```python
from build123d import *

# Parameters (mm, degrees)
SKETCH1_R      = 2.15
EXTRUDE1_DEPTH = 3


with BuildPart() as part:
    # Sketch1 → Extrude1 (new body)
    with BuildSketch(Plane.XY):
        Polygon((-85, 225.999923245), (-85, 210.999923245), (-55, 180.999923245), (-40, 180.999923245), (-26, 194.999923245), (26, 194.999923245), (40, 180.999923245), (55, 180.999923245), (85, 210.999923245), (85, 225.999923245), align=None)
        with Locations((-47.5, 188.999923245)):
            Circle(SKETCH1_R, mode=Mode.SUBTRACT)
        with Locations((-47.5, 203.999923245)):
            Circle(SKETCH1_R, mode=Mode.SUBTRACT)
        with Locations((-75, 218.499923245)):
            Circle(SKETCH1_R, mode=Mode.SUBTRACT)
        with Locations((-20, 218.499923245)):
            Circle(SKETCH1_R, mode=Mode.SUBTRACT)
        with Locations(Location((47.5, 188.999923245, 0), (0, 0, 180))):
            Circle(SKETCH1_R, mode=Mode.SUBTRACT)
        with Locations(Location((47.5, 203.999923245, 0), (0, 0, 180))):
            Circle(SKETCH1_R, mode=Mode.SUBTRACT)
        with Locations(Location((20, 218.499923245, 0), (0, 0, 180))):
            Circle(SKETCH1_R, mode=Mode.SUBTRACT)
        with Locations(Location((75, 218.499923245, 0), (0, 0, 180))):
            Circle(SKETCH1_R, mode=Mode.SUBTRACT)
    extrude(amount=EXTRUDE1_DEPTH)


solid = part.part
```
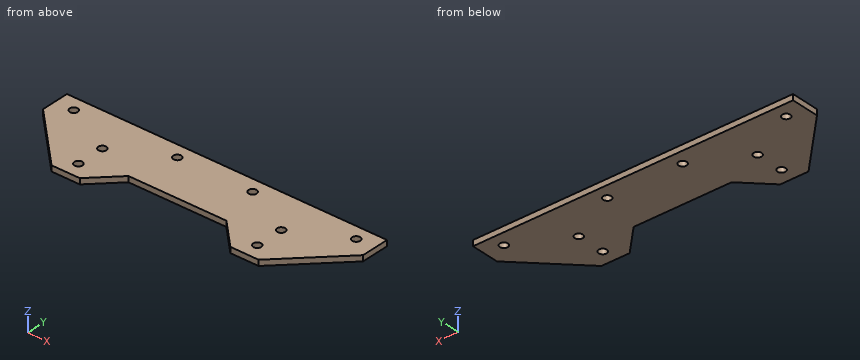
CAD build for the part. Positions are in the model's coordinates, mm. Give positions to 0.01 mm unless a question says otherwise; leave off trailing zeros. Write each loop counter-clockwise with the first axis right and the second up, starting at its lowest first coordinate (ties: lowest second). Pieces come first, ordered by that corner, then holes. Notation, with made-up numbers: (75, 63.5) -> (110, 63.5) arc R12 cw to (110, 72.5) -> close; hole circle Ø6 at (-8.75, 76). An arc over 180 degrees is marked (long way). Write each question's results on one line, items separated by ' | '.
1. Cut at D-D, the plane x = 75. Write the cut outline in (y, z), then the cut area to 3 significant figures.
Geometry check:
outline: (201, 0) -> (216.35, 0) -> (216.35, 3) -> (201, 3) -> close; (220.65, 0) -> (226, 0) -> (226, 3) -> (220.65, 3) -> close | area: 62.1 mm²
2. Cut at C-C, the plane z = 0.7. Give the number of separate pieces and of enclosed holes in the cut face, then the cut area to 3 significant figures.
Geometry check:
separate pieces: 1 | enclosed holes: 8 | area: 5,710 mm²
3. Cut at B-B, the plane x = -47.5. Write the cut outline in (y, z), then the cut area to 3 significant figures.
Geometry check:
outline: (181, 0) -> (186.85, 0) -> (186.85, 3) -> (181, 3) -> close; (191.15, 0) -> (201.85, 0) -> (201.85, 3) -> (191.15, 3) -> close; (206.15, 0) -> (226, 0) -> (226, 3) -> (206.15, 3) -> close | area: 109 mm²
4. Cut at A-A, the plane x = -20. Write the cut outline in (y, z).
Geometry check:
outline: (195, 0) -> (216.35, 0) -> (216.35, 3) -> (195, 3) -> close; (220.65, 0) -> (226, 0) -> (226, 3) -> (220.65, 3) -> close
5. Drop flat-ended pins along their axis: P1, Ø4, axis at x = -47.5, y = 189, coming from the -Z side (3 decimals); P2, Ø1.5, axis at x = -1, z = 2, coming from the -Y side. Give the stop position or say it passes through.
Geometry check:
P1: through | P2: y = 195
6. Wall check: probe 1 along Y at (x, z) = (-47.5, 1.75); probe 2 along Y at (x, z) = (-20, 2); probe 3 along X at (y, z) = (219, 1.95). Give the ranges that are in metal, low to high. Write a range as [from, to].
Geometry check:
probe 1: [181, 186.85], [191.15, 201.85], [206.15, 226] | probe 2: [195, 216.35], [220.65, 226] | probe 3: [-85, -77.09], [-72.91, -22.09], [-17.91, 17.91], [22.09, 72.91], [77.09, 85]
